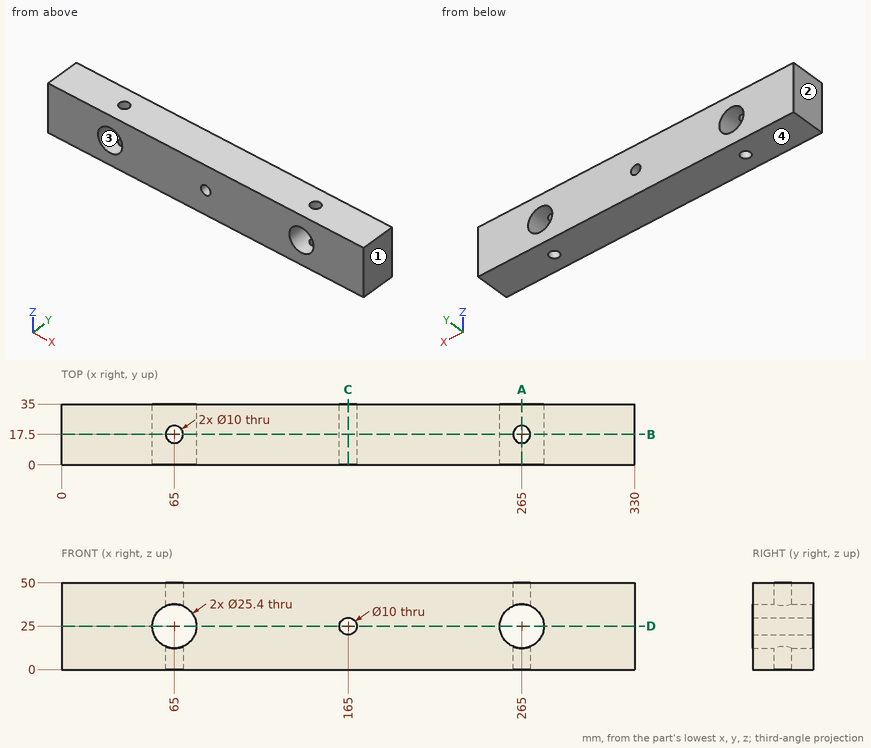
Verification items for this drawing (mm, ordinates from the low corner). Round coordinates to 2 decimals unless told otherwise and drop trailing zeros. Write each loop counter-clockwise with the first axis right and the second up, starting at its lowest first coordinate (ties: lowest second). Pieces come first, ordered by that corner, then holes. Notation, with made-up numbers: M 32,40 L 45,40 A28 cw 45,67 Z; hole C -16,15 d6. An arc over 180 degrees is marked long. Write item = value, one per line. Start each with the question number.
1. Section check D-D, the plane z = 25. Record the cut outline in (x, y).
2. Section check B-B, the plane y = 17.5. Record the cut outline in (x, z).
3. Release check for a two-part mould opening along X. For the marked faces 1, 2, 3 and 4 record: pulls with the +X half, pulls with the -X half, needs draft (parallel to the pull), parting line crosses it, or undercut.
4. Section check C-C, the plane x = 165. Record the cut outline in (y, z).
5. Scan lines: line 1 (X direction, y = 17, z = 46); line 2 (X direction, y = 28, z = 27); line 3 (Z direction, x = 165.5, y = 6). Record each from-to range of solid material in increasing order. Write a range as [from, to].
6. Section check A-A, the plane x = 265. Record the cut outline in (y, z).
7. Gauge pin test, flat end, axial feed: pin 1 (8 mm diameter, centred on x = 165, z = 25, fed in from -Y). Record the tip position at first contact, or that the pin passes through.
Results found:
q1.outline = M 0,0 L 52.3,0 L 52.3,35 L 0,35 Z; M 77.7,0 L 160,0 L 160,35 L 77.7,35 Z; M 170,0 L 252.3,0 L 252.3,35 L 170,35 Z; M 277.7,0 L 330,0 L 330,35 L 277.7,35 Z
q2.outline = M 0,0 L 60,0 L 60,13.33 A12.7 cw 60,36.67 L 60,50 L 0,50 Z; M 70,0 L 260,0 L 260,13.33 A12.7 cw 260,36.67 L 260,50 L 70,50 L 70,36.67 A12.7 cw 70,13.33 Z; M 270,0 L 330,0 L 330,50 L 270,50 L 270,36.67 A12.7 cw 270,13.33 Z; hole C 165,25 d10
q3.face_1 = pulls with the +X half
q3.face_2 = pulls with the -X half
q3.face_3 = undercut
q3.face_4 = needs draft
q4.outline = M 0,0 L 35,0 L 35,20 L 0,20 Z; M 0,30 L 35,30 L 35,50 L 0,50 Z
q5.line_1 = [0, 60.03], [69.97, 260.03], [269.97, 330]
q5.line_2 = [0, 52.46], [77.54, 160.42], [169.58, 252.46], [277.54, 330]
q5.line_3 = [0, 20.03], [29.97, 50]
q6.outline = M 0,0 L 12.5,0 L 12.5,12.3 L 0,12.3 Z; M 0,37.7 L 12.5,37.7 L 12.5,50 L 0,50 Z; M 22.5,0 L 35,0 L 35,12.3 L 22.5,12.3 Z; M 22.5,37.7 L 35,37.7 L 35,50 L 22.5,50 Z
q7.pin_1 = through
